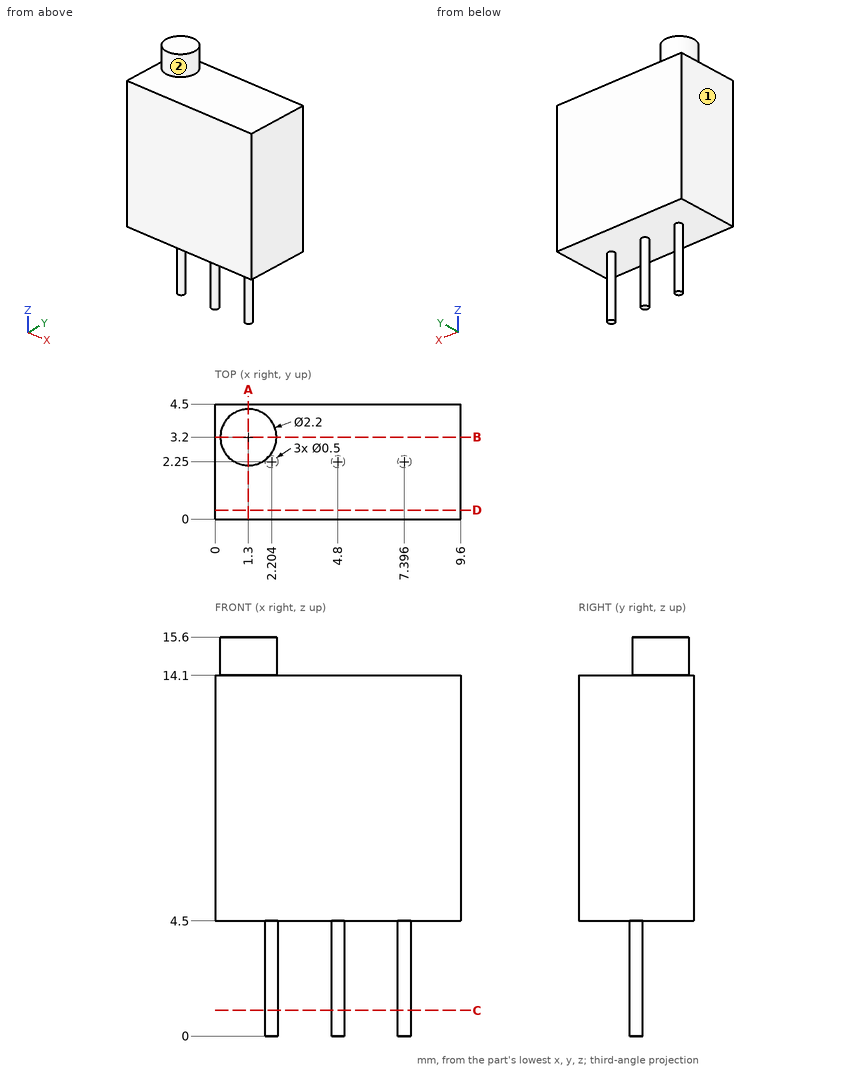
Design review of the part shown in the three views and the two pictorial views. Dimensions are in mm from the part's minimum x, y and z. A direction names the side the tool comes from. Coordinates: 2 decimals unless noted, no trailing zeros. Loops run counter-clockwise (first coordinate to the right, second up) from the corner with the lowest first, then second, coordinate; pieces in that order, holes last.
Q1. We need section B-B on y = 3.2. State the section outline as (x, z) points.
Reported:
outline: (0, 4.5) - (9.6, 4.5) - (9.6, 14.1) - (2.4, 14.1) - (2.4, 15.6) - (0.2, 15.6) - (0.2, 14.1) - (0, 14.1) - close
Q2. We need section C-C on z = 1. State the section outline as (x, y) points, and give its area (3 significant figures).
Reported:
outline: circle Ø0.5 at (2.2, 2.25); circle Ø0.5 at (4.8, 2.25); circle Ø0.5 at (7.4, 2.25)
area: 0.589 mm2
Q3. We need section A-A on x = 1.3. State the section outline as (y, z) points.
Reported:
outline: (0, 4.5) - (4.5, 4.5) - (4.5, 14.1) - (4.3, 14.1) - (4.3, 15.6) - (2.1, 15.6) - (2.1, 14.1) - (0, 14.1) - close
Q4. To check wall thickness, follow line 1 (Z direction, x = 6.75, y = 0.7); line 2 (Z direction, x = 1.5, y = 3.65); line 3 (Y direction, x = 4.75, z = 2) (3 decimals). State the ranges of each line that lie inside material, in increasing order.
Reported:
line 1: z = 4.5 to 14.1
line 2: z = 4.5 to 15.6
line 3: y = 2.005 to 2.495
Q5. We need section D-D on y = 0.35. State the section outline as (x, z) points.
Reported:
outline: (0, 4.5) - (9.6, 4.5) - (9.6, 14.1) - (0, 14.1) - close
Q6. Tool access review of the marked faces 1 and 2: name each direction out of +Z, -Z, +X, -X, +Y, -Y from which nothing blocks a thin tool from reaching the whole face with its end or side.
Reported:
face 1: +Z, -Z, -X, +Y, -Y
face 2: +Z
Q7. For pin 1 (2 mm diameter, centred on x = 5.5, y = 1, fed in from -Z), flat-tipped, find the tip position at first contact; note if it passes through.
Reported:
pin 1: stops at z = 4.5
